from build123d import *

# Parameters (mm, degrees)
F0_W     = 44.45
F0_H     = 33.3248
F1_DEPTH = 7.9375
F2_W     = 25.4
F2_H     = 25.4
F3_DEPTH = 12.7
F5_W     = 12.7
F5_H     = 19.05
F6_DEPTH = 3.176
F7_R     = 6.34999
F8_W     = 12.7
F8_H     = 6.35
F9_DEPTH = 12.7
F11_D    = 4.4958
F13_D    = 3.4544


# Not quite as in the source:
# - a fillet or chamfer is up to 0.001 mm smaller than in the source, because OpenCascade refuses the exact size
# - a pattern or mirror of a feature is missing from the dataset's text; its kind, count and spacing are read off the source's solid


with BuildPart() as f1:
    # F0 (on Front) → F1 (new body, symmetric)
    with BuildSketch(Plane.XZ):
        with Locations((0, 16.6624)):
            Rectangle(F0_W, F0_H)
    extrude(amount=F1_DEPTH, both=True)

    # F2 (on face) → F3 (cut)
    with BuildSketch(Plane.XZ.offset(7.9375)):
        with Locations((0, 20.6248)):
            Rectangle(F2_W, F2_H)
    extrude(amount=-F3_DEPTH, mode=Mode.SUBTRACT)

    # F5 (on face) → F6 (cut, through all)
    with BuildSketch(Plane.XZ.offset(-4.7625)):
        with Locations((0, 23.7998)):
            Rectangle(F5_W, F5_H)
    extrude(amount=-F6_DEPTH, mode=Mode.SUBTRACT)

    # F7 (radius 6.35 in the source; OpenCascade refuses exactly that, so slightly less here)
    f7_edges = [f1.edges().sort_by_distance(p)[0] for p in [
        (-6.35, 6.35, 14.2748),
        (6.35, 6.35, 14.2748),
    ]]
    fillet(f7_edges, radius=F7_R)

    # F8 (on face) → F9 (join)
    with BuildSketch(Plane(origin=(-22.225, 0, 0), x_dir=(0, -1, 0), z_dir=(-1, 0, 0))):
        with Locations((14.2875, 3.175)):
            Rectangle(F8_W, F8_H)
    f9 = extrude(amount=-F9_DEPTH)

    # F9_copies: F9 across plane
    add(f9.mirror(Plane(origin=(0, 0, 0), x_dir=(0, 0, 1), z_dir=(1, 0, 0))))

    # F11 (through all)
    with Locations(Plane.XY.offset(6.35)):
        with Locations((-15.875, -14.2875)):
            f11 = Hole(F11_D / 2)

    # F11_copies: F11 across plane
    add(f11.mirror(Plane(origin=(0, 0, 0), x_dir=(0, 0, 1), z_dir=(1, 0, 0))), mode=Mode.SUBTRACT)

    # F13 (through all)
    with Locations(Plane(origin=(-22.225, 0, 0), x_dir=(0, -1, 0), z_dir=(-1, 0, 0))):
        with Locations((1.5875, 20.6248)):
            Hole(F13_D / 2)


solid = f1.part
For this review, take the finished solid that the model builds, in its own axes (mm). A direction names the side the tool comes from. Give positions to 0.01 mm unless a question says otherwise; leave off trailing zeros. Order: outer loops, then holes, each group sorted by start corner. A loop starts at its lowest first (then second) coordinate and runs counter-clockwise, first axis right, second up. Notation, with made-up numbers: (6, 88) - (45, 88) arc R27 cw to (45, 124) - close; hole circle Ø7 at (-8, 21). An arc over 180 degrees is marked (long way). Answer as a JSON object with one key per item and string values. Group by question number.
Item 1: Machinability: for faces 1 (the cylindrical face through (-4.539, 6.372, 16.184)), 2 (the flat face through (-6, 4.762, 18)), 3 (the flat face through (-9.525, -14, 3)), 4 (the flat face through (-16, -11, 6.35)), which of the approach directions +Z, -Z, +X, -X, +Y, -Y give a long, thin tool a straight path to every point of the face, cutting with its end or side? Answer none if there is none.
Item 2: Clearance check with flat-ended pins moving along their axes: pin 1 Ø7 at (x, y) = (-15.88, -14.29) entering from +Z; pin 2 Ø4 at (y, z) = (-10, 19) entering from +X; pin 3 Ø7.5 at (x, z) = (-1.5, 15) entering from -Y; pin 4 Ø5 at (x, z) = (12, 20) entering from -Y. State where each tip first meets the part, or that it passes through.
Item 3: Take a section at D-D on x = -17. Give the boundary of the cut face in (y, z).
Item 4: Take a section at B-B on x = 19.5. Give the boundary of the cut face in (y, z), and give its area (3 significant figures).
Item 5: Wall thickness on line 1 along X through (y, z) = (2.5, 15) (3 decimals); line 2 along Z through (x, y) = (-11.5, 0.75); line 3 along Z through (x, y) = (-16, -16.75): over which ranges is each line inside the solid? List them lowest first.
Item 6: Take a section at C-C on y = -1. Give the boundary of the cut face in (x, z) (3 decimals), and give its area (3 significant figures).
Item 7: Draft analysis for pull direction Y (two halves, no side actions). For faces 5 (the cylindrical face through (17.95, -15.15, 3.13)), 6 (the cylindrical face through (-17.95, -15.15, 3.13)), 7 (the flat face through (0, 7.938, 13)), 8 (the flat face through (6.35, 6, 27)), state which applies: pulls with the +Y half, pulls with the -Y half, needs draft (parallel to the pull), parting line crosses it, or undercut.
Reported:
{
 "1": {"face 1": "+Z, +Y, -Y", "face 2": "+Z, -Y", "face 3": "+Z, -Z, -Y", "face 4": "+Z, +X, -X, -Y"},
 "2": {"pin 1": "z = 6.35", "pin 2": "through", "pin 3": "y = 4.76", "pin 4": "y = -7.94"},
 "3": {"outline": "(-20.64, 0) - (-16.23, 0) - (-16.23, 6.35) - (-20.64, 6.35) - close; (-12.34, 0) - (7.94, 0) - (7.94, 33.32) - (-7.94, 33.32) - (-7.94, 6.35) - (-12.34, 6.35) - close; hole circle Ø3.45 at (-1.59, 20.62)"},
 "4": {"outline": "(-20.64, 0) - (7.94, 0) - (7.94, 33.32) - (-7.94, 33.32) - (-7.94, 6.35) - (-20.64, 6.35) - close; hole circle Ø3.45 at (-1.59, 20.62)", "area": "600 mm^2"},
 "5": {"line 1": "-22.225 to -12.7, 12.7 to 22.225", "line 2": "0 to 7.92", "line 3": "0 to 6.35"},
 "6": {"outline": "(-22.225, 0) - (22.225, 0) - (22.225, 19.001) - (12.7, 19.001) - (12.7, 7.925) - (-12.7, 7.925) - (-12.7, 19.001) - (-22.225, 19.001) - close; (-22.225, 22.249) - (-12.7, 22.249) - (-12.7, 33.325) - (-22.225, 33.325) - close; (12.7, 22.249) - (22.225, 22.249) - (22.225, 33.325) - (12.7, 33.325) - close", "area": "774 mm^2"},
 "7": {"face 5": "undercut", "face 6": "undercut", "face 7": "pulls with the +Y half", "face 8": "needs draft"}
}
